Here's how the part is built. I have some questions about the finished solid (model axes, mm). Face numbers are marked on the shaded views. A direction names the side the tool comes from. Coordinates: 2 decimals unless noted, no trailing zeros. Loops run counter-clockwise (first coordinate to the right, second up) from the corner with the lowest first, then second, coordinate; pieces in that order, holes last. Notation, with made-up numbers: M 73.25,1 L 108.25,1 A19 cw 108.25,12 Z; hole C 62.5,52.25 d10. An arc over 180 degrees is marked long. Use CSV: the item, a comma, the result in double quotes. Start each with the question number.
Q1. For pin 1 Ø12 at (y, z) = (-14, -33) entering from +X; pin 2 Ø12 at (y, z) = (2, -30) entering from +X; pin 3 Ø14.5 at (y, z) = (4, -11) entering from -X; pin 4 Ø7 at (x, y) = (31, 0) entering from -Z, each with a flat end and sliding along its axis, tell me the tip position at first contact or that it passes through.
Q2. If we section it at C-C (y = -10.5): Please give me the cut outline in (x, z).
Q3. Please list where these lines run through material, in increasing order: probe 1 along Y at (x, z) = (-31, -21); probe 2 along Y at (x, z) = (0, -35); probe 3 along Z at (x, y) = (40.5, 5.5). Write a range as [from, to].
Q4. If we mould it in two halves opening along Y, with no side actions, what happens to the marked faces 4, 5 and 6? For each: +Y half, -Y half, draft (parallel to the pull), parting line (faces both ways), or undercut.
Q5. If we section it at D-D (z = -32.5): Please give me the cut outline in (x, y), and give its area (3 significant figures).
Q6. If we section it at B-B (z = -17): Please give me the cut outline in (x, y), and give its area (3 significant figures).
Q7. If we section it at A-A (x = 0): Please give me the cut outline in (y, z).
Q8. Which directions (+Z, -Z, +X, -X, +Y, -Y) give clear straight access to the entire face, cutting with the end or side of a thin tool? Please do the marked faces 1, 2 and 3.
from build123d import *

# Parameters (mm, degrees)
BOSS_EXTRUDE1_DEPTH = 18
CUT_EXTRUDE1_DEPTH  = 36
SKETCH7_R           = 4.5
CUT_EXTRUDE3_DEPTH  = 36
CUT_EXTRUDE4_DEPTH  = 11


with BuildPart() as part:
    # Sketch2 → Boss-Extrude1 (new body, symmetric)
    with BuildSketch(Plane(origin=(0, 0, 0), x_dir=(1, 0, 0), z_dir=(0, 1, 0))):
        with BuildLine():
            Line((-25.690465157, 28), (-50, 28))
            Line((-50, 28), (-50, 19))
            Line((-50, 19), (-21.027756377, 19))
            Line((-21.027756377, 19), (-21.027756377, 6))
            Line((-21.027756377, 6), (-18.027756377, 6))
            ThreePointArc((-18.027756377, 6), (0, 19), (18.027756377, 6))
            Line((18.027756377, 6), (21.027756377, 6))
            Line((21.027756377, 6), (21.027756377, 19))
            Line((21.027756377, 19), (50, 19))
            Line((50, 19), (50, 28))
            Line((50, 28), (25.690465157, 28))
            ThreePointArc((25.690465157, 28), (0, 38), (-25.690465157, 28))
        make_face()
    extrude(amount=BOSS_EXTRUDE1_DEPTH, both=True)

    # Sketch4 → Cut-Extrude1 (cut)
    with BuildSketch(Plane(origin=(0, 0, -28), x_dir=(-1, 0, 0), z_dir=(0, 0, -1))):
        with BuildLine():
            Line((-50, -18), (-44.497190923, -18))
            ThreePointArc((-44.497190923, -18), (-48, 0), (-44.497190923, 18))
            Line((-44.497190923, 18), (-50, 18))
            Line((-50, 18), (-50, -18))
        make_face()
    cut_extrude1 = extrude(amount=-CUT_EXTRUDE1_DEPTH, mode=Mode.SUBTRACT)

    # Mirror1: Cut-Extrude1 across plane
    add(cut_extrude1.mirror(Plane(origin=(0, 0, 0), x_dir=(0, 0, 1), z_dir=(1, 0, 0))), mode=Mode.SUBTRACT)

    # Sketch7 → Cut-Extrude3 (cut)
    with BuildSketch(Plane(origin=(0, 0, -28), x_dir=(-1, 0, 0), z_dir=(0, 0, -1))):
        with Locations((-31, 0)):
            Circle(SKETCH7_R)
    cut_extrude3 = extrude(amount=-CUT_EXTRUDE3_DEPTH, mode=Mode.SUBTRACT)

    # Sketch8 → Cut-Extrude4 (cut, through all)
    with BuildSketch(Plane(origin=(0, 0, -28), x_dir=(-1, 0, 0), z_dir=(0, 0, -1))):
        with BuildLine():
            Line((-25.690465157, 6.637683312), (-25.690465157, -6.637683312))
            ThreePointArc((-25.690465157, -6.637683312), (-22.5, 0), (-25.690465157, 6.637683312))
        make_face()
    cut_extrude4 = extrude(amount=CUT_EXTRUDE4_DEPTH, mode=Mode.SUBTRACT)

    # Mirror3: Cut-Extrude3, Cut-Extrude4 across plane
    add(cut_extrude3.mirror(Plane(origin=(0, 0, 0), x_dir=(0, 0, 1), z_dir=(1, 0, 0))), mode=Mode.SUBTRACT)
    add(cut_extrude4.mirror(Plane(origin=(0, 0, 0), x_dir=(0, 0, 1), z_dir=(1, 0, 0))), mode=Mode.SUBTRACT)

    # Sketch11 → CBORE for M5 Hex Head Bolt1 (revolve, cut)
    with BuildSketch(Plane(origin=(0, 0, -38), x_dir=(0, 1, 0), z_dir=(1, 0, 0))):
        Polygon((0, 0), (0, 32), (2.5, 32), (2.5, 13.300129879), (2.9995, 13), (3, 0), align=None)
    revolve(axis=Axis((0, 0, -44.35), (0, 0, 1)), mode=Mode.SUBTRACT)


solid = part.part
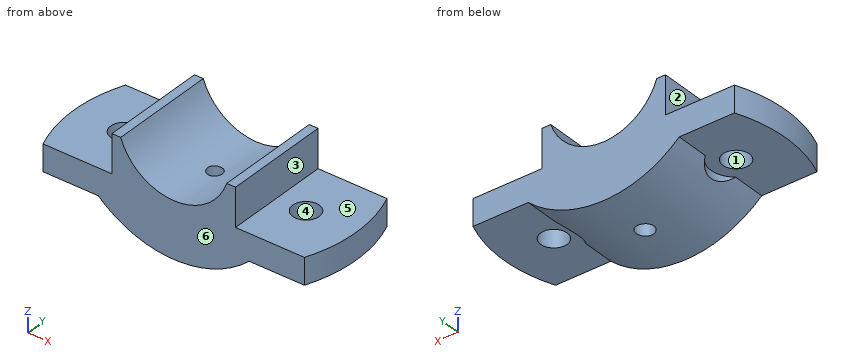
Results below:
1,pin 1,"x = 46.8"
1,pin 2,"x = 48"
1,pin 3,"x = -21.03"
1,pin 4,"through"
2,outline,"M -46.84,-28 L -25.69,-28 A38 ccw 25.69,-28 L 46.84,-28 L 46.84,-19 L 21.03,-19 L 21.03,-6 L 18.03,-6 A19 cw -18.03,-6 L -21.03,-6 L -21.03,-19 L -46.84,-19 Z"
3,probe 1,"[-18, -4.5], [4.5, 18]"
3,probe 2,"[-18, -3], [3, 18]"
3,probe 3,"[-28, -19]"
4,face 4,"undercut"
4,face 5,"draft"
4,face 6,"-Y half"
5,outline,"M -19.69,-18 L 19.69,-18 L 19.69,18 L -19.69,18 Z; hole C 0,0 d6"
5,area,"1,390 mm^2"
6,outline,"M -21.03,-18 L -8.49,-18 L -8.49,18 L -21.03,18 Z; M 8.49,-18 L 21.03,-18 L 21.03,18 L 8.49,18 Z"
6,area,"903 mm^2"
7,outline,"M -18,-38 L -3,-38 L -3,-25 L -2.5,-24.7 L -2.5,-19 L -18,-19 Z; M 2.5,-24.7 L 3,-25 L 3,-38 L 18,-38 L 18,-19 L 2.5,-19 Z"
8,face 1,"+Z, -Z"
8,face 2,"+Z, -X, +Y, -Y"
8,face 3,"+Z, +X, +Y, -Y"
